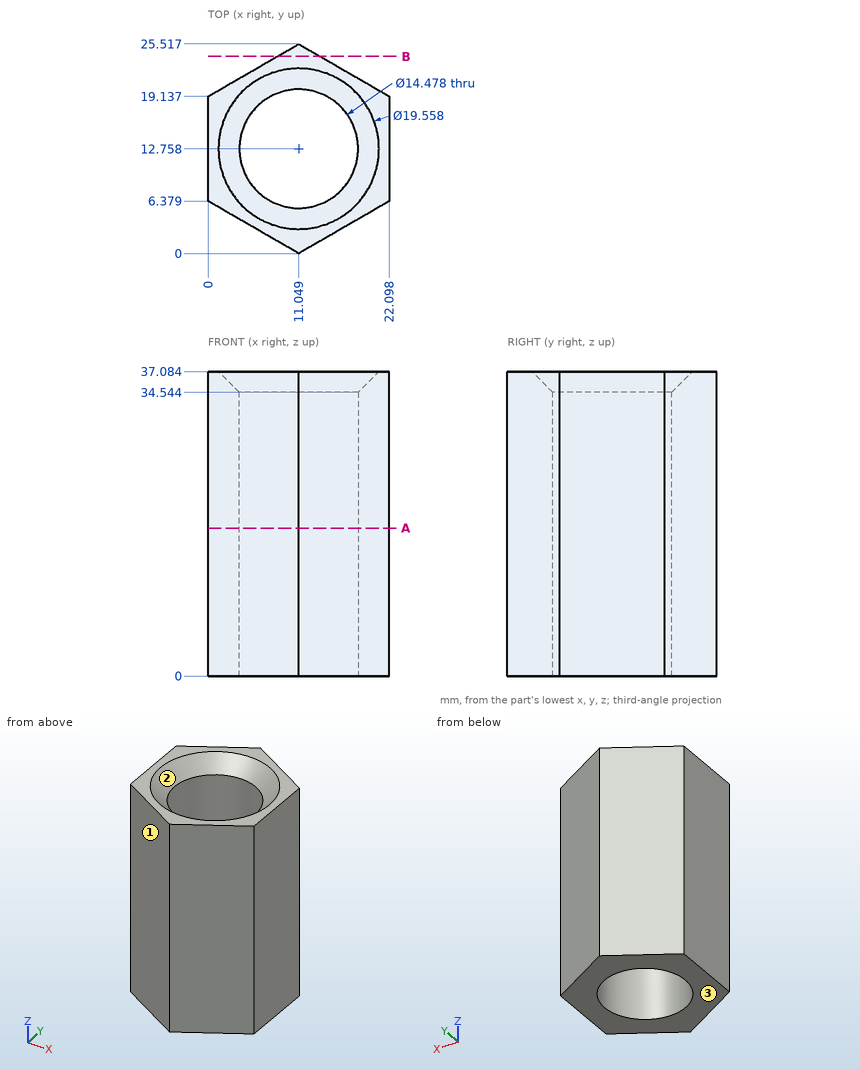
Geometry: see drawing. Coordinates: mm, zero at the bounding-box minimum. Coordinates: 2 decimals unless noted, no trailing zeros. Loops run counter-clockwise (first coordinate to the right, second up) from the corner with the lowest first, then second, coordinate; pieces in that order, holes last. Notation, with made-up numbers: (51.25, -18) - (80.25, -18) arc R18 ccw to (80.25, 14) - close; hole circle Ø5 at (-10, 72). An arc over 180 degrees is marked (long way). Put each result on its own line as item: value. Start each with the question number.
Q1. Cut plane A-A, the plane z = 18. Return loops of the section in (x, y).
Q2. Pin query (flat end, axial travel): pin 1 Ø10 at (x, z) = (6.5, 9.5) entering from +Y; pin 2 Ø8.5 at (x, y) = (11.05, 12.76) entering from -Z; pin 3 Ø1.5 at (y, z) = (23, 22.5) entering from +X (1 decimal); pin 4 Ø4 at (x, z) = (11.5, 21) entering from -Y. Return the tip coordinate at first contact, or that it passes through.
Q3. Cut plane B-B, the plane y = 24. Return loops of the section in (x, z) (1 decimal).
Q4. Line query: line 1 (X direction, y = 11.25, z = 24); line 2 (X direction, y = 12.5, z = 10) (1 decimal); line 3 (Y direction, x = 14.5, z = 14.5) (1 decimal). Output: solid intervals per line, ascending.
Q5. Pull-direction query (X, two-part tool) for the marked faces 1, 2 and 3; classes: released by +X, released by -X, zero draft, split by the parting line, or undercut.
Filled sheet:
1. outline: (0, 6.38) - (11.05, 0) - (22.1, 6.38) - (22.1, 19.14) - (11.05, 25.52) - (0, 19.14) - close; hole circle Ø14.48 at (11.05, 12.76)
2. pin 1: y = 25.52
2. pin 2: through
2. pin 3: x = 16.7
2. pin 4: y = 0
3. outline: (8.4, 0) - (13.7, 0) - (13.7, 37.1) - (8.4, 37.1) - close
4. line 1: 0 to 3.97, 18.13 to 22.1
4. line 2: 0 to 3.8, 18.3 to 22.1
4. line 3: 2 to 6.4, 19.1 to 23.5
5. face 1: released by -X
5. face 2: undercut
5. face 3: zero draft
